CAD build for the part. Positions are in the model's coordinates, mm. Face numbers are marked on the shaded views. A direction names the side the tool comes from. Give positions to 0.01 mm unless a question says otherwise; leave off trailing zeros. Order: outer loops, then holes, each group sorted by start corner. A loop starts at its lowest first (then second) coordinate and runs counter-clockwise, first axis right, second up. Notation, with made-up numbers: (-19.5, -15.75) -> (28.5, -15.75) arc R24 ccw to (28.5, 21.25) -> close; hole circle Ø6 at (34, 52.5). An arc over 180 degrees is marked (long way). Answer as CSV lines item,"result".
```python
from build123d import *

# Parameters (mm, degrees)
F1_DEPTH = 7.5
F2_R     = 5
F3_R     = 1.5
F4_DEPTH = 5
F5_R     = 1.5
F6_DEPTH = 5


with BuildPart() as f1:
    # F0 (on Front) → F1 (new body, symmetric)
    with BuildSketch(Plane.XZ):
        Polygon((-3, 5), (-5, 5), (-5, -5), (5, -5), (5, -3), (-3, -3), align=None)
    extrude(amount=F1_DEPTH, both=True)

    # F2
    f2_edges = [f1.edges().sort_by_distance(p)[0] for p in [
        (-4, -7.5, 5),
        (-4, 7.5, 5),
        (5, -7.5, -4),
        (5, 7.5, -4),
    ]]
    fillet(f2_edges, radius=F2_R)

    # F3 (on Right) → F4 (cut)
    with BuildSketch(Plane.YZ):
        with Locations((-2.5, 0)):
            Circle(F3_R)
        with Locations((2.5, 0)):
            Circle(F3_R)
    extrude(amount=-F4_DEPTH, mode=Mode.SUBTRACT)

    # F5 (on Top) → F6 (cut)
    with BuildSketch(Plane.XY):
        with Locations((0, 2.5)):
            Circle(F5_R)
        with Locations((0, -2.5)):
            Circle(F5_R)
    extrude(amount=-F6_DEPTH, mode=Mode.SUBTRACT)


solid = f1.part
```
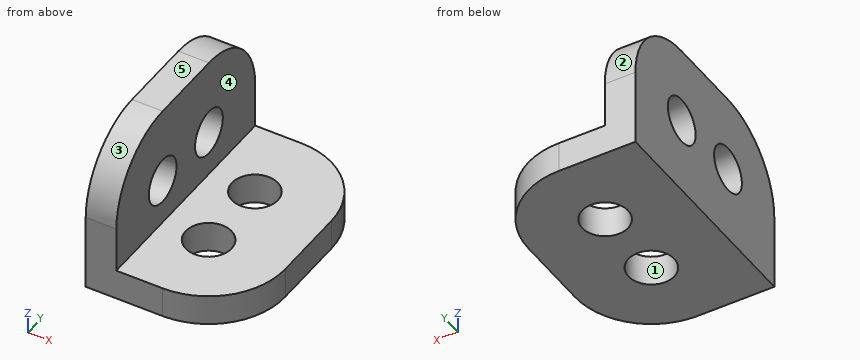
1) Band-saw the part on D-D, the plane y = 0. Write the cut outline in (x, z), then the cut area to 3 significant figures.
Data:
outline,"(-5, -5) -> (5, -5) -> (5, -3) -> (-3, -3) -> (-3, 5) -> (-5, 5) -> close"
area,"36.0 mm2"
2) Pull direction Y, two halves, no side cores. Call the marked faces 1, 2 and 3: pulls with the +Y half, pulls with the -Y half, needs draft (parallel to the pull), parting line crosses it, or undercut.
Data:
face 1,"undercut"
face 2,"pulls with the +Y half"
face 3,"pulls with the -Y half"
3) Which spindle directions (+Z, -Z, +X, -X, +Y, -Y) get a long thin tool onto all of the face, cutting with end or side? Do the marked faces 4 and 5. Say none if no direction does.
Data:
face 4,"+Z, +X, +Y, -Y"
face 5,"+Z, +X, -X, +Y, -Y"
4) Band-saw the part on B-B, the plane y = -3.5. Write the cut outline in (x, z).
Data:
outline,"(-5, -5) -> (-1.12, -5) -> (-1.12, -3) -> (-3, -3) -> (-3, -1.12) -> (-5, -1.12) -> close; (-5, 1.12) -> (-3, 1.12) -> (-3, 4.9) -> (-5, 4.9) -> close; (1.12, -5) -> (4.9, -5) -> (4.9, -3) -> (1.12, -3) -> close"
5) Band-saw the part on C-C, the plane x = -0.25. Write the cut outline in (y, z), then the cut area to 3 significant figures.
Data:
outline,"(-7.5, -5) -> (-3.98, -5) -> (-3.98, -3) -> (-7.5, -3) -> close; (-1.02, -5) -> (1.02, -5) -> (1.02, -3) -> (-1.02, -3) -> close; (3.98, -5) -> (7.5, -5) -> (7.5, -3) -> (3.98, -3) -> close"
area,"18.2 mm2"
6) Wall check: line 1 along Z through (x, y) = (-4.45, -2.5); line 2 along Z through (x, y) = (-2.5, -3.5). Give the ranges that are in metal, low to high. Write a range as [from, to].
Data:
line 1,"z = [-5, -1.5], [1.5, 5]"
line 2,"z = [-5, -3]"
7) Band-saw the part on A-A, the plane z = -3.25. Write the cut outline in (x, y).
Data:
outline,"(-5, -7.5) -> (0, -7.5) arc R5 ccw to (5, -2.5) -> (5, 2.5) arc R5 ccw to (0, 7.5) -> (-5, 7.5) -> close; hole circle Ø3 at (0, -2.5); hole circle Ø3 at (0, 2.5)"
8) Pin check, flat tips, straight feed: P1, Ø4, axis at x = 0, y = -2.5, coming from the +Z side; P2, Ø4, axis at y = -5.5, z = 1, coming from the +X side; P3, Ø1.5, axis at x = 2.5, z = -0.5, coming from the -Y side. Stop position of each tip, or through.
Data:
P1,"stops at z = -3"
P2,"stops at x = -3"
P3,"passes through"
